```python
from build123d import *

# Parameters (mm, degrees)
SKETCH1_R                = 1
BOSS_EXTRUDE1_DEPTH      = 1
FILLET1_R                = 3
SKETCH2_R                = 2
BOSS_EXTRUDE2_DEPTH      = 0.1
BOSS_EXTRUDE2_DEPTH_BACK = 1.1
SKETCH3_R                = 1
CUT_EXTRUDE1_DEPTH       = 2
SKETCH4_W                = 2.5
SKETCH4_H                = 2
SKETCH4_W_2              = 1
BOSS_EXTRUDE3_DEPTH      = 1


with BuildPart() as part:
    # Sketch1 → Boss-Extrude1 (new body)
    with BuildSketch(Plane.XY):
        with BuildLine():
            Line((11, 4), (11, -4))
            ThreePointArc((11, -4), (14, -7), (11, -10))
            Line((11, -10), (-4, -10))
            ThreePointArc((-4, -10), (-14, 0), (-4, 10))
            Line((-4, 10), (11, 10))
            ThreePointArc((11, 10), (14, 7), (11, 4))
        make_face()
        with Locations((12, 7)):
            Circle(SKETCH1_R, mode=Mode.SUBTRACT)
        with Locations((12, -7)):
            Circle(SKETCH1_R, mode=Mode.SUBTRACT)
    extrude(amount=BOSS_EXTRUDE1_DEPTH)

    # Fillet1
    fillet1_edges = [part.edges().sort_by_distance(p)[0] for p in [
        (11, 4, 0.5),
        (11, -4, 0.5),
    ]]
    fillet(fillet1_edges, radius=FILLET1_R)

    # Sketch2 → Boss-Extrude2 (add, two sides)
    with BuildSketch(Plane.XY.offset(1)) as boss_extrude2_sk:
        with Locations((12, 7)):
            Circle(SKETCH2_R)
        with Locations((12, -7)):
            Circle(SKETCH2_R)
    extrude(amount=BOSS_EXTRUDE2_DEPTH)
    extrude(boss_extrude2_sk.sketch, amount=-BOSS_EXTRUDE2_DEPTH_BACK)

    # Sketch3 → Cut-Extrude1 (cut)
    with BuildSketch(Plane.XY.offset(1.1)):
        with Locations((12, 7)):
            Circle(SKETCH3_R)
        with Locations((12, -7)):
            Circle(SKETCH3_R)
    extrude(amount=-CUT_EXTRUDE1_DEPTH, mode=Mode.SUBTRACT)

    # Sketch4 → Boss-Extrude3 (add)
    with BuildSketch(Plane.XY.offset(1)):
        with Locations((8.25, 2)):
            Rectangle(SKETCH4_W, SKETCH4_H)
        with Locations((7.7, -1.5)):
            Rectangle(SKETCH4_W_2, SKETCH4_H)
        with Locations((7, -6.25)):
            Rectangle(SKETCH4_W_2, SKETCH4_H)
    extrude(amount=BOSS_EXTRUDE3_DEPTH)


solid = part.part
```
CAD build for the part. Positions are in the model's coordinates, mm. A direction names the side the tool comes from. Coordinates: 2 decimals unless noted, no trailing zeros. Loops run counter-clockwise (first coordinate to the right, second up) from the corner with the lowest first, then second, coordinate; pieces in that order, holes last. Notation, with made-up numbers: (85.5, 27) - (114.5, 27) arc R20 cw to (114.5, 41) - close; hole circle Ø9 at (16.25, 7). An arc over 180 degrees is marked (long way). Return JSON: item names as keys, results as strings.
1. Band-saw the part on B-B (x = 12). State how many separate pieces and enclosed holes the cut face has, and give its area (3 significant figures).
Result:
{"separate pieces": "4", "enclosed holes": "0", "area": "8.38 mm2"}
2. Probe L1, parallel to Y at x = 12, z = 0.3; L2, parallel to Z at x = 9.25, y = -2; L3, parallel to Y at x = 6.75, z = 1.2. List the from-to ranges inside material, lowest first. Write a range as from..to.
Result:
{"L1": "y = -9.83..-8, -6..-4.04, 4.04..6, 8..9.83", "L2": "z = 0..1", "L3": "y = -7.25..-5.25"}
3. Band-saw the part on A-A (z = 0.45). Give the cut face in (x, y).
Result:
{"outline": "(-4, -10) - (11, -10) arc R3 ccw to (12.5, -4.4) arc R3 cw to (11, -1.8) - (11, 1.8) arc R3 cw to (12.5, 4.4) arc R3 ccw to (11, 10) - (-4, 10) arc R10 ccw to start; hole circle Ø2 at (12, -7); hole circle Ø2 at (12, 7)"}
4. Band-saw the part on C-C (x = 8.5). Give the cut face in (y, z).
Result:
{"outline": "(-10, 0) - (10, 0) - (10, 1) - (3, 1) - (3, 2) - (1, 2) - (1, 1) - (-10, 1) - close"}
5. Band-saw the part on D-D (y = 0). Give the cut face in (x, z), and give its area (3 significant figures).
Result:
{"outline": "(-14, 0) - (11, 0) - (11, 1) - (-14, 1) - close", "area": "25.0 mm2"}
6. Drop flat-ended pins along their axis: pin 1 (0.5 mm diameter, centred on y = 2, z = 1.5, fed in from +X); pin 2 (10 mm diameter, centred on x = -0.5, y = -4.5, fed in from -Z); pin 3 (4.5 mm diameter, centred on x = 11.5, y = 8, fed in from +Z). Give the stop position or say it passes through.
Result:
{"pin 1": "stops at x = 9.5", "pin 2": "stops at z = 0", "pin 3": "stops at z = 1.1"}
7. 3-axis set-ups, long thin cutter, end or side, ignore diameter. For faces 1 (the flat face through (8.2, 3, 1.5)), 2 (the flat face through (6.5, -6.3, 1.5)), 3 (the flat face through (7, 2, 1.5)): which of +Z, -Z, +X, -X, +Y, -Y reach the whole face in a straight line?
Result:
{"face 1": "+Z, +X, -X, +Y", "face 2": "+Z, -X, +Y, -Y", "face 3": "+Z, -X, +Y"}
